Part model, mm, in its own coordinate system. Give positions to 0.01 mm unless a question says otherwise; leave off trailing zeros. Order: outer loops, then holes, each group sorted by start corner. A loop starts at its lowest first (then second) coordinate and runs counter-clockwise, first axis right, second up. Notation, with made-up numbers: (22.25, 88.25) - (60.25, 88.25) arc R18 cw to (60.25, 116.25) - close; hole circle Ø4 at (-24.75, -15). An arc over 180 degrees is marked (long way). One line per item, written item: value.
```python
from build123d import *

# Parameters (mm, degrees)
SKETCH2_R           = 2.5
BOSS_EXTRUDE1_DEPTH = 5
SKETCH5_R           = 2.5
BOSS_EXTRUDE2_DEPTH = 5
SCALE1_SCALE        = 0.6


with BuildPart() as part:
    # Sketch2 → Boss-Extrude1 (new body)
    with BuildSketch(Plane.XY):
        with BuildLine():
            Line((-3.705099972, 4.386006173), (-2.28681669, -3.158891918))
            ThreePointArc((-2.28681669, -3.158891918), (0, -5.055887715), (2.28681669, -3.158891918))
            Line((2.28681669, -3.158891918), (3.705099972, 4.386006173))
            ThreePointArc((3.705099972, 4.386006173), (0, 8.852481252), (-3.705099972, 4.386006173))
        make_face()
        with Locations((0, 5.082487595)):
            Circle(SKETCH2_R, mode=Mode.SUBTRACT)
    extrude(amount=BOSS_EXTRUDE1_DEPTH)

    # Sketch5 → Boss-Extrude2 (add)
    with BuildSketch(Plane.XY.offset(5)):
        with Locations(Location((0, -1.656861976, 0), (0, 0, 180))):
            Circle(SKETCH5_R)
    extrude(amount=BOSS_EXTRUDE2_DEPTH)


with BuildPart() as part_1:
    # Scale1: scaled about (0, 0, 0)
    add(part.part.scale(SCALE1_SCALE))


solid = part_1.part
```
1) Cut at D-D, the plane x = 1.1. Give the cut face in (y, z).
Outcome:
outline: (-2.5, 0) - (2.03, 0) - (2.03, 3) - (0.03, 3) - (0.03, 6) - (-2.01, 6) - (-2.01, 3) - (-2.5, 3) - close; (4.07, 0) - (5.03, 0) - (5.03, 3) - (4.07, 3) - close
2) Drill centre lines: line 1 along Z through (x, y) = (1.65, 1); line 2 along Y through (x, z) = (1.25, 2.25); line 3 along Y through (x, z) = (-0.5, 4.6). Where is each one in solid material? Low to high. Write a range as from..to.
Outcome:
line 1: z = 0..3
line 2: y = -2.26..2.22, 3.88..4.93
line 3: y = -2.41..0.42
3) Cut at A-A, the plane x = 0. Give the cut face in (y, z), then the cut area to 3 significant figures.
Outcome:
outline: (-3.03, 0) - (1.55, 0) - (1.55, 3) - (0.51, 3) - (0.51, 6) - (-2.49, 6) - (-2.49, 3) - (-3.03, 3) - close; (4.55, 0) - (5.31, 0) - (5.31, 3) - (4.55, 3) - close
area: 25.0 mm^2
4) Pin check, flat tips, straight feed: pin 1 (2.5 mm diameter, centred on x = 0, y = 2, fed in from +Z); pin 2 (3 mm diameter, centred on y = -2, z = 5, fed in from -X). Stop position of each tip, or through.
Outcome:
pin 1: stops at z = 3
pin 2: stops at x = -1.5
5) Cut at C-C, the plane z = 1.5. Give the cut face in (x, y), then the cut area to 3 significant figures.
Outcome:
outline: (-2.22, 2.63) - (-1.37, -1.9) arc R1.4 ccw to (1.37, -1.9) - (2.22, 2.63) arc R2.26 ccw (long way) to start; hole circle Ø3 at (0, 3.05)
area: 21.5 mm^2
6) Mould opens along Y. For faces 1 (the cylindrical face through (-1.431, -1.445, 4.479)), 2 (the flat face through (0, 1, 3)), 3 (the flat face through (1.792, 0.336, 1.479)), 4 (the cylindrical face through (-0.325, 1.585, 1.479)) say: released by +Y, released by -Y, zero draft, split by the parting line, or undercut.
Outcome:
face 1: split by the parting line
face 2: zero draft
face 3: released by -Y
face 4: undercut
7) Cut at B-B, the plane y = 3.5. Give the cut face in (x, z), then the cut area to 3 significant figures.
Outcome:
outline: (-2.22, 0) - (-1.43, 0) - (-1.43, 3) - (-2.22, 3) - close; (1.43, 0) - (2.22, 0) - (2.22, 3) - (1.43, 3) - close
area: 4.72 mm^2
